Can you work these out from the model? Positions are in its coordinate system, mm. Face numbers are marked on the shaded views. A direction names the side the tool comes from. Coordinates: 2 decimals unless noted, no trailing zeros. Loops run counter-clockwise (first coordinate to the right, second up) from the corner with the lowest first, then second, coordinate; pieces in that order, holes last. Notation, with made-up numbers: (58.5, -27.75) -> (87.5, -27.75) arc R10 cw to (87.5, -16.75) -> close; hole circle Ø11 at (62, 45). An arc over 180 degrees is marked (long way). Put each result on its own line as item: value. Start each with the question number.
Item 1: If we section it at A-A on x = 0: Please give me the cut outline in (y, z), plus the area to 3 significant figures.
Item 2: Will these pins go through, and if not, where does the flat tip stop? P1, Ø7.5, axis at y = -19, z = -12.5, coming from the +X side; P2, Ø6.5, axis at x = 60.5, y = -10.5, coming from the -Z side; P3, Ø13, axis at x = -56.5, y = -38, coming from the -Z side; P4, Ø16.5, axis at x = 0, z = 4.23, coming from the +Y side.
Item 3: Please list where these lines run through material, in increasing order: L1, parallel to Z at x = 0, y = -18.5; L2, parallel to X at y = -26, z = -7.5; L3, parallel to Y at x = 15.5, z = 23. Write a range as from..to.
Item 4: We'd pull the mould along X, two halves only. Please class the marked faces 4, 5 and 6: pulls with the +X half, pulls with the -X half, needs draft (parallel to the pull), parting line crosses it, or undercut.
Item 5: If we section it at B-B on y = -16: Please give me the cut outline in (x, z), plus the area to 3 significant figures.
Item 6: If we section it at D-D on z = -3.5: Please give me the cut outline in (x, y).
Item 7: For the marked faces 1, 2 and 3, which set-ups out of +Z, -Z, +X, -X, +Y, -Y let a thin tool reach every point of the face, with its end or its side?
Item 8: If we section it at C-C on z = 29: Please give me the cut outline in (x, y).
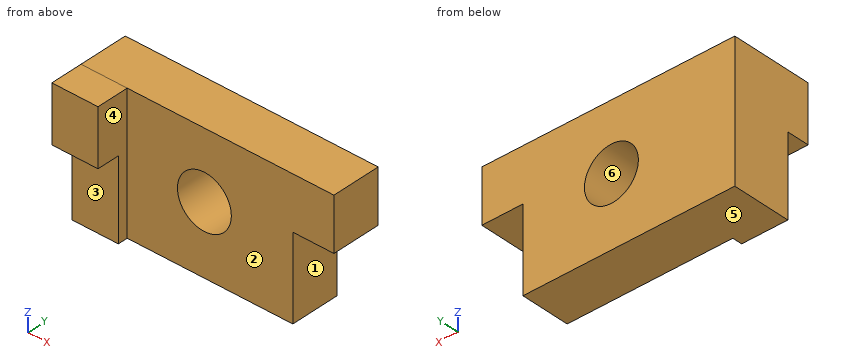
```python
from build123d import *

# Parameters (mm, degrees)
F0_W     = 130.872465
F0_H     = 70.537049
F0_R     = 13.948248
F1_DEPTH = 25.4
F2_W     = 21.569185
F2_H     = 43.13836
F3_DEPTH = 40.386
F4_W     = 23.900985
F4_H     = 41.389507
F5_DEPTH = 30.48
F6_W     = 23.900985
F6_H     = 29.147542
F7_DEPTH = 42.164


with BuildPart() as f1:
    # F0 (on Front) → F1 (new body)
    with BuildSketch(Plane.XZ):
        with Locations((1.603116, 3.643444)):
            Rectangle(F0_W, F0_H)
        with Locations((0, 4.226394)):
            Circle(F0_R, mode=Mode.SUBTRACT)
    extrude(amount=F1_DEPTH)

    # F2 (on Front) → F3 (cut)
    with BuildSketch(Plane.XZ):
        with Locations((56.546229, -10.055901)):
            Rectangle(F2_W, F2_H)
    extrude(amount=F3_DEPTH, mode=Mode.SUBTRACT)

    # F4 (on Front) → F5 (join)
    with BuildSketch(Plane.XZ):
        with Locations((-51.882624, -10.930327)):
            Rectangle(F4_W, F4_H)
    extrude(amount=F5_DEPTH)

    # F6 (on Front) → F7 (join)
    with BuildSketch(Plane.XZ):
        with Locations((-51.882624, 24.338197)):
            Rectangle(F6_W, F6_H)
    extrude(amount=F7_DEPTH)


solid = f1.part
```
Solutions:
1. outline: (-25.4, -31.63) -> (0, -31.63) -> (0, -9.72) -> (-25.4, -9.72) -> close; (-25.4, 18.17) -> (0, 18.17) -> (0, 38.91) -> (-25.4, 38.91) -> close
1. area: 1,080 mm^2
2. P1: x = 45.76
2. P2: z = 11.51
2. P3: z = 9.76
2. P4: through
3. L1: -31.63..-9.72, 18.17..38.91
3. L2: -63.83..-39.93
3. L3: -25.4..0
4. face 4: pulls with the +X half
4. face 5: needs draft
4. face 6: undercut
5. outline: (-63.83, -31.63) -> (45.76, -31.63) -> (45.76, 11.51) -> (67.04, 11.51) -> (67.04, 38.91) -> (-63.83, 38.91) -> close; hole circle Ø27.9 at (0, 4.23)
5. area: 7,700 mm^2
6. outline: (-63.83, -30.48) -> (-39.93, -30.48) -> (-39.93, -25.4) -> (-11.61, -25.4) -> (-11.61, 0) -> (-63.83, 0) -> close; (11.61, -25.4) -> (45.76, -25.4) -> (45.76, 0) -> (11.61, 0) -> close
7. face 1: -Z, +X, +Y, -Y
7. face 2: +Z, -Z, +X, -Y
7. face 3: -Z, +X, -X, -Y
8. outline: (-63.83, -42.16) -> (-39.93, -42.16) -> (-39.93, -25.4) -> (67.04, -25.4) -> (67.04, 0) -> (-63.83, 0) -> close
